Here's how the part is built. I have some questions about the finished solid (model axes, mm). A direction names the side the tool comes from. Coordinates: 2 decimals unless noted, no trailing zeros. Write each loop counter-clockwise with the first axis right and the second up, starting at its lowest first coordinate (ties: lowest second). Pieces come first, ordered by that corner, then holes.
(1) Imagine slicing it at C-C, the plane x = 0. State how many separate pieces and enclosed holes the cut face has, plus the area to 3 significant figures.
(2) Imagine slicing it at B-B, the plane z = 22. List the corners of the cut face in (x, y) for me, plus the area to 3 significant figures.
(3) For pin 1 Ø8 at (x, y) = (16, -15.5) entering from -Z; pin 2 Ø1 at (x, z) = (16, 24.5) entering from +Y; pin 3 Ø17 at (x, y) = (-11.5, 2) entering from -Z; pin 4 Ø2 at (y, z) = (-8, 20.5) entering from -X, each with a flat end and sliding along its axis, tell me the tip position at first contact or that it passes through.
(4) Thinking about a two-plate mould opening in Z: for faces 1 (the cylindrical face through (-9.29, 3.27, 36.86)), 2 (the flat face through (-5.7, 20.5, 44.284)), 3 (the flat face through (23, 15, 34.784)), which applies, released by +Z, released by -Z, zero draft, split by the parting line, or undercut?
(5) Imagine slicing it at A-A, the plane z = 40. List the corners of the cut face in (x, y) for me (1 decimal), plus the area to 3 significant figures.
(6) Please list where these lines run through material, in increasing order: probe 1 along Y at (x, z) = (0, 36); probe 2 along Y at (x, z) = (-12, 33); probe 3 along Y at (x, z) = (0, 41.9).
(7) Which directions (+Z, -Z, +X, -X, +Y, -Y) give clear straight access to the entire face, cutting with the end or side of a thin tool? Please do faces 4 (the cylindrical face through (-26.36, 5.85, 23.29)), 5 (the cylindrical face through (-4.336, -19.524, 42.79)), 6 (the flat face through (11.787, -9.103, 36.86)).
Autodesk Inventor part; units mm, degrees
ref_plane "Work Plane1" through (0, 0, 29.2835) normal (0, 0, -1) x (-1, 0, 0)
ref_plane "YZ Plane" through (0, 0, 0) normal (1, 0, 0) x (0, 1, 0)
ref_plane "XZ Plane" through (0, 0, 0) normal (0, 1, 0) x (-1, 0, 0)
sketch "Sketch1" plane through (0, 0, 0) normal (0, 1, 0) x (-1, 0, 0)
  line L0 (0, 0) -> (0, 48.3347) construction
  line L1 (-23, 44.2835) -> (-28, 44.2835)
  line L2 (-28, 44.2835) -> (-28, 14.2835)
  line L3 (-28, 14.2835) -> (-23, 14.2835)
  line L4 (-23, 14.2835) -> (-23, 44.2835)
  point P0 (0, 23.2008)
  dimension "d2" = 5
  dimension "d3" = 30
  dimension "d4" = 23
revolve "Revolution1" add sketch "Sketch1" angle 360 about axis through (0, 0, 0) along (0, 0, 1)
sketch "Sketch7" plane through (0, 0, 44.2835) normal (0, 0, 1) x (1, 0, 0)
  circle A0 centre (0, 0) radius 24
  dimension "d33" = 48
extrude "Extrusion4" add sketch "Sketch7" against normal blind 13
fillet "Fillet4" radius 3 2 edges at (-28, 0, 44.2835) (-28, 0, 14.2835)
sketch "Sketch8" plane through (0, 0, 44.2835) normal (0, 0, 1) x (1, 0, 0)
  circle A0 centre (0, 0) radius 23
  circle A1 centre (0, 0) radius 25
  circle A2 centre (0, 0) radius 28
  circle A3 centre (0, 0) radius 25
  circle A4 centre (0, 0) radius 23
fillet "Fillet5" radius 3 1 edges at (-23, 0, 31.2835)
sketch "Sketch9" plane through (0, 0, 44.2835) normal (0, 0, 1) x (1, 0, 0)
  circle A0 centre (0, 0) radius 23
  circle A1 centre (0, 0) radius 20
  circle A2 centre (0, 0) radius 20
extrude "Extrusion5" cut sketch "Sketch9" against normal blind 2 contours A1
chamfer "Chamfer1" distance 1 angle 45 1 edges at (-20, 0, 44.2835)
sketch "Sketch10" plane through (0, 0, 42.2835) normal (0, 0, 1) x (1, 0, 0)
  line L0 (-16.9268, -6.6619) -> (-10.5367, -4.6226)
  line L1 (-6.7299, -12.6441) -> (-4.1467, -7.8856)
  arc A0 (-16.9268, -6.6619) -> (-6.7299, -12.6441) centre (-7.1975, -1.7595) ccw
  arc A1 (-10.5367, -4.6226) -> (-4.1467, -7.8856) centre (7.1055, 22.0383) ccw
  point P0 (0, 0)
extrude "Extrusion6" cut sketch "Sketch10" against normal through all
pattern_circular "Circular Pattern2" count 6 over 360 about axis through (0, 0, -10) along (0, 0, 1) of "Extrusion6"
sketch "Sketch11" plane through (0, 0, 42.2835) normal (0, 0, 1) x (1, 0, 0)
  point P0 (0, 0)
hole "Hole3" at (0, 0, 44.2835) direction (0, 0, -1) diameter 3.2 end through all counterbore diameter 10 counterbore depth 3
sketch "Sketch12" plane through (0, 0, 31.2835) normal (0, 0, -1) x (-1, 0, 0)
  point P0 (0, 0)
hole "Hole4" at (0, 0, 31.2835) direction (0, 0, 1) diameter 3.2 end through all counterbore diameter 10 counterbore depth 2
sketch "Sketch13" plane through (0, 0, 0) normal (1, 0, 0) x (0, 1, 0)
  line L0 (-28, 17.2835) -> (-28, 41.2835)
  line L1 (-28, 39.2835) -> (-27, 39.2835)
  line L2 (-27, 39.2835) -> (-27, 38.2835)
  line L3 (-27, 38.2835) -> (-28, 38.2835)
  line L4 (-28, 38.2835) -> (-28, 39.2835)
  line L5 (-28, 35.7835) -> (-27, 35.7835)
  line L6 (-27, 35.7835) -> (-27, 34.7835)
  line L7 (-27, 34.7835) -> (-28, 34.7835)
  line L8 (-28, 34.7835) -> (-28, 35.7835)
  line L9 (-28, 32.2835) -> (-27, 32.2835)
  line L10 (-27, 32.2835) -> (-27, 31.2835)
  line L11 (-27, 31.2835) -> (-28, 31.2835)
  line L12 (-28, 31.2835) -> (-28, 32.2835)
  line L13 (-28, 41.2835) -> (-28, 17.2835) construction
  arc A0 (-28, 17.2835) -> (-25, 14.2835) centre (-25, 17.2835) ccw construction
  line L14 (-28, 17.2835) -> (28, 17.2835) construction
  line L15 (-28, 29.2835) -> (28, 29.2835) construction
  line L16 (0, -8.8567) -> (0, 53.1402)
  point P0 (0, 0)
  dimension "d62" = 1
  dimension "d63" = 1
  dimension "d64" = 1
  dimension "d65" = 1
  dimension "d66" = 1
  dimension "d67" = 1
  dimension "d68" = 10
  dimension "d69" = 2.5
  dimension "d70" = 2.5
revolve "Revolution2" cut sketch "Sketch13" angle 360 about axis through (0, 0, -10) along (0, 0, 1)
ref_plane "Work Plane1" through (0, 0, 29.2835) normal (0, 0, -1) x (-1, 0, 0)
mirror "Mirror1" about plane through (0, 0, 29.2835) normal (0, 0, -1) of "Revolution2"
properties part number "Wheels1" material "ABS Plastic"
Recorded:
1. separate pieces: 4
1. enclosed holes: 0
1. area: 591 mm2
2. outline: circle Ø56 at (0, 0); hole circle Ø46 at (0, 0)
2. area: 801 mm2
3. pin 1: stops at z = 14.28
3. pin 2: stops at y = 23.32
3. pin 3: stops at z = 31.28
3. pin 4: stops at x = -27.11
4. face 1: zero draft
4. face 2: released by +Z
4. face 3: undercut
5. outline: circle Ø56 at (0, 0); hole (-16.9, -6.7) arc R10.9 ccw to (-6.7, -12.6) - (-4.1, -7.9) arc R32 cw to (-10.5, -4.6) - close; hole (-14.3, -0.5) - (-8.9, -0.4) arc R32 cw to (-9.3, 6.8) - (-14.2, 11.3) arc R10.9 ccw to start; hole (-7.6, 12.2) - (-4.8, 7.5) arc R32 cw to (1.3, 11.4) - (2.7, 18) arc R10.9 ccw to start; hole (-2.7, -18) arc R10.9 ccw to (7.6, -12.2) - (4.8, -7.5) arc R32 cw to (-1.3, -11.4) - close; hole circle Ø3.2 at (0, 0); hole (4.1, 7.9) arc R32 cw to (10.5, 4.6) - (16.9, 6.7) arc R10.9 ccw to (6.7, 12.6) - close; hole (8.9, 0.4) arc R32 cw to (9.3, -6.8) - (14.2, -11.3) arc R10.9 ccw to (14.3, 0.5) - close
5. area: 2,080 mm2
6. probe 1: y = -28 to -17.81, -10.77 to -1.6, 1.6 to 10.77, 17.81 to 28
6. probe 2: y = -25.3 to -11.54, -5.09 to -0.43, 9.3 to 25.3
6. probe 3: y = -27.94 to -17.81, -10.77 to -5, 5 to 10.77, 17.81 to 27.94
7. face 4: none
7. face 5: +Z
7. face 6: +Z, -Z
